from build123d import *

# Parameters (mm, degrees)
BASE_FLANGE1_DEPTH = 1
FILLET1_R          = 2
SKETCH6_R          = 1.5
CUT_EXTRUDE1_DEPTH = 97.006984786


# Sheet-metal steps are written as plain solids
with BuildPart() as part:
    # Sketch1 → Base-Flange1 (new body)
    with BuildSketch(Plane.XY):
        Polygon((-38.5, 0), (38.5, 0), (36, 40), (30, 52), (30, 88), (-30, 88), (-30, 52), (-36, 40), align=None)
    extrude(amount=-BASE_FLANGE1_DEPTH)

    # Fillet1
    fillet1_edges = [part.edges().sort_by_distance(p)[0] for p in [
        (38.5, 0, -0.5),
        (-38.5, 0, -0.5),
        (-36, 40, -0.5),
        (-30, 52, -0.5),
        (-30, 88, -0.5),
        (30, 88, -0.5),
        (30, 52, -0.5),
        (36, 40, -0.5),
    ]]
    fillet(fillet1_edges, radius=FILLET1_R)

    # Sketch6 → Cut-Extrude1 (cut, through all)
    with BuildSketch(Plane.XY):
        with Locations((-25, 82)):
            Circle(SKETCH6_R)
        with Locations((25, 82)):
            Circle(SKETCH6_R)
        with Locations((-25, 47)):
            Circle(SKETCH6_R)
        with Locations((25, 47)):
            Circle(SKETCH6_R)
        with Locations((-29.5, 5)):
            Circle(SKETCH6_R)
        with Locations((28.5, 5)):
            Circle(SKETCH6_R)
    extrude(amount=-CUT_EXTRUDE1_DEPTH, mode=Mode.SUBTRACT)


solid = part.part
Geometry: final body of the model. Coordinates: model frame, mm. Round coordinates to 2 decimals unless told otherwise and drop trailing zeros. Loops run counter-clockwise (first coordinate to the right, second up) from the corner with the lowest first, then second, coordinate; pieces in that order, holes last. Notation, with made-up numbers: (77.25, -29.75) - (133.25, -29.75) arc R18 ccw to (133.25, -2.75) - close; hole circle Ø8 at (47, 6.25). An arc over 180 degrees is marked (long way). Write each question's results on one line, items separated by ' | '. Start each with the question number.
1) Line query: probe 1 along X at (y, z) = (82, -0.4); probe 2 along Y at (x, z) = (-25, -0.7); probe 3 along X at (y, z) = (59, -0.5). Output: solid intervals per line, ascending. Write a range as [from, to].
2) Cut plane B-B on z = -0.65. Return loops of the section in (x, y).
3) First-contact query: P1, Ø4, axis at x = -25, y = 47, coming from the +Z side; P2, Ø1.8, axis at x = -29.5, y = 5, coming from the +Z side; P3, Ø0.5, axis at y = 63, z = -0.5, coming from the -X side. Flat tips, straight axial feed; report the tip coordinate or a pass-through.
4) Cut plane D-D on y = 68. Return loops of the section in (x, z).
5) Cut plane A-A on y = 82. Return loops of the section in (x, z).
6) Cut plane C-C on x = 25. Return loops of the section in (y, z), then the cut area to 3 significant figures.
Verdict:
1) probe 1: x = [-30, -26.5], [-23.5, 23.5], [26.5, 30] | probe 2: y = [0, 45.5], [48.5, 80.5], [83.5, 88] | probe 3: x = [-30, 30]
2) outline: (-38.37, 2.12) arc R2 ccw to (-36.37, 0) - (36.37, 0) arc R2 ccw to (38.37, 2.12) - (36.03, 39.59) arc R2 ccw to (35.82, 40.36) - (30.21, 51.58) arc R2 cw to (30, 52.47) - (30, 86) arc R2 ccw to (28, 88) - (-28, 88) arc R2 ccw to (-30, 86) - (-30, 52.47) arc R2 cw to (-30.21, 51.58) - (-35.82, 40.36) arc R2 ccw to (-36.03, 39.59) - close; hole circle Ø3 at (-29.5, 5); hole circle Ø3 at (-25, 47); hole circle Ø3 at (-25, 82); hole circle Ø3 at (25, 47); hole circle Ø3 at (25, 82); hole circle Ø3 at (28.5, 5)
3) P1: stops at z = 0 | P2: passes through | P3: stops at x = -30
4) outline: (-30, -1) - (30, -1) - (30, 0) - (-30, 0) - close
5) outline: (-30, -1) - (-26.5, -1) - (-26.5, 0) - (-30, 0) - close; (-23.5, -1) - (23.5, -1) - (23.5, 0) - (-23.5, 0) - close; (26.5, -1) - (30, -1) - (30, 0) - (26.5, 0) - close
6) outline: (0, -1) - (45.5, -1) - (45.5, 0) - (0, 0) - close; (48.5, -1) - (80.5, -1) - (80.5, 0) - (48.5, 0) - close; (83.5, -1) - (88, -1) - (88, 0) - (83.5, 0) - close | area: 82.0 mm2
